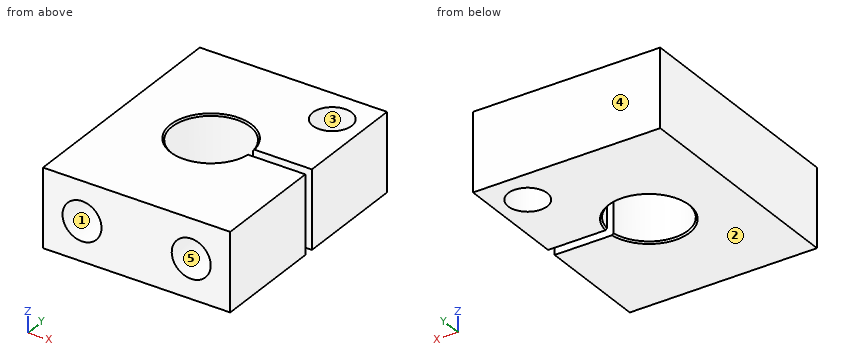
from build123d import *

# Parameters (mm, degrees)
SKETCH1_W           = 30.48
SKETCH1_H           = 38.1
BOSS_EXTRUDE1_DEPTH = 6.35
CUT_EXTRUDE2_DEPTH  = 13.7
CHAMFER1_SIZE       = 0.254
SKETCH8_R           = 3.175
CUT_EXTRUDE4_DEPTH  = 13.7


with BuildPart() as part:
    # Sketch1 → Boss-Extrude1 (new body, symmetric)
    with BuildSketch(Plane.XY):
        Rectangle(SKETCH1_W, SKETCH1_H)
    extrude(amount=BOSS_EXTRUDE1_DEPTH, both=True)

    # Sketch2 → Cut-Extrude2 (cut, through all)
    with BuildSketch(Plane.XY.offset(6.35)):
        with BuildLine():
            Line((97.980767498, 0.79375), (15.24, 0.79375))
            Line((15.24, 0.79375), (5.665195309, 0.79375))
            ThreePointArc((5.665195309, 0.79375), (-6.985, 0), (5.665195309, -0.79375))
            Line((5.665195309, -0.79375), (15.24, -0.79375))
            Line((15.24, -0.79375), (97.980767498, -0.79375))
            Line((97.980767498, -0.79375), (263.462302495, -0.79375))
            Line((263.462302495, -0.79375), (263.462302495, 0.79375))
            Line((263.462302495, 0.79375), (97.980767498, 0.79375))
        make_face()
    extrude(amount=-CUT_EXTRUDE2_DEPTH, mode=Mode.SUBTRACT)

    # Sketch6 → 1/4 (0.25) Diameter Hole1 (revolve, cut)
    with BuildSketch(Plane(origin=(8.89, -19.05, 0), x_dir=(0, 0, -1), z_dir=(1, 0, 0))):
        Polygon((0, 0), (0, 9.527732465), (3.175, 7.62), (3.175, 0), align=None)
    f_1_4_0_25_diameter_hole1 = revolve(axis=Axis((8.89, -25.4, 0), (0, 1, 0)), mode=Mode.SUBTRACT)

    # Chamfer1
    chamfer1_edges = [part.edges().sort_by_distance(p)[0] for p in [
        (-6.985, 0, -6.35),
        (-6.985, 0, 6.35),
    ]]
    chamfer(chamfer1_edges, length=CHAMFER1_SIZE)

    # Mirror1: 1/4 (0.25) Diameter Hole1 across plane
    add(f_1_4_0_25_diameter_hole1.mirror(Plane(origin=(0, 0, 0), x_dir=(0, 0, 1), z_dir=(1, 0, 0))), mode=Mode.SUBTRACT)

    # Sketch8 → Cut-Extrude4 (cut, through all)
    with BuildSketch(Plane.XY.offset(6.35)):
        with Locations((10.16, 13.335)):
            Circle(SKETCH8_R)
    extrude(amount=-CUT_EXTRUDE4_DEPTH, mode=Mode.SUBTRACT)


solid = part.part
Geometry check sheet. Reference: the model listing, model coordinates, mm. Face numbers are marked on the shaded views. A direction names the side the tool comes from. Round coordinates to 2 decimals unless told otherwise and drop trailing zeros. Order: outer loops, then holes, each group sorted by start corner. A loop starts at its lowest first (then second) coordinate and runs counter-clockwise, first axis right, second up. Notation, with made-up numbers: M 51,15.25 L 58,15.25 A23 cw 58,50.25 Z; hole C -15.75,44 d6. An arc over 180 degrees is marked long. Answer in a Markdown table with one row per item.
(1) Sectioned sample at B-B, the plane y = 12. Record the cut outline in (x, z).
Responses:
| item | result |
|---|---|
| outline | M -15.24,-6.35 L 7.28,-6.35 L 7.28,6.35 L -15.24,6.35 Z; M 13.04,-6.35 L 15.24,-6.35 L 15.24,6.35 L 13.04,6.35 Z |
(2) Go/stop test with a flat-tipped pin: P1, Ø5, axis at x = 8.89, z = 0, coming from the -Y side. Record where the tip stops, or that it passes through.
Responses:
| item | result |
|---|---|
| P1 | stops at y = -11.02 |
(3) Draft check along Y on the marked faces 3, 4 and 5. Enter one of: released by +Y, released by -Y, zero draft, split by the parting line, or undercut.
Responses:
| item | result |
|---|---|
| face 3 | undercut |
| face 4 | released by +Y |
| face 5 | zero draft |
(4) Tool access check on the marked faces 1 and 2. Record the directions out of +Z, -Z, +X, -X, +Y, -Y that give a thin tool (end or side, any length) a straight path to the whole face; none if there is none.
Responses:
| item | result |
|---|---|
| face 1 | -Y |
| face 2 | -Z, +X, -X, +Y, -Y |
(5) Sectioned sample at C-C, the plane y = 0. Record the cut outline in (x, z) (3 decimals), and give its area (3 significant figures).
Responses:
| item | result |
|---|---|
| outline | M -15.24,-6.35 L -7.239,-6.35 L -6.985,-6.096 L -6.985,6.096 L -7.239,6.35 L -15.24,6.35 Z |
| area | 105 mm² |
(6) Sectioned sample at D-D, the plane x = 11.5. State how many separate pieces and enclosed holes the cut face has, and give its area (3 significant figures).
Responses:
| item | result |
|---|---|
| separate pieces | 3 |
| enclosed holes | 0 |
| area | 362 mm² |
(7) Scan lines: probe 1 along X at (y, z) = (-13.75, 0) (3 decimals); probe 2 along Y at (x, z) = (6, 4.25); probe 3 along X at (y, z) = (-15.5, -2). Record each from-to range of solid material in increasing order. Write a range as from..to.
Responses:
| item | result |
|---|---|
| probe 1 | x = -15.24..-12.065, -5.715..5.715, 12.065..15.24 |
| probe 2 | y = -19.05..-0.79, 0.79..19.05 |
| probe 3 | x = -15.24..-11.36, -6.42..6.42, 11.36..15.24 |
(8) Sectioned sample at A-A, the plane z = 4. Record the cut outline in (x, y) (3 decimals).
Responses:
| item | result |
|---|---|
| outline | M -15.24,-19.05 L 15.24,-19.05 L 15.24,-0.794 L 5.665,-0.794 A6.35 cw long 5.665,0.794 L 15.24,0.794 L 15.24,19.05 L -15.24,19.05 Z; hole C 10.16,13.335 d6.35 |
